Input: part model. Units: mm. Frame: model coordinates. A direction names the side the tool comes from. Round coordinates to 2 decimals unless told otherwise and drop trailing zeros. Loops run counter-clockwise (first coordinate to the right, second up) from the corner with the lowest first, then second, coordinate; pieces in that order, holes last. Notation, with made-up numbers: M 53.25,-6.5 L 82.25,-6.5 A11 cw 82.25,3.5 Z; hole C 51.5,0 d4. An arc over 180 degrees is marked long. Return JSON: item names as keys, results as strings. Group by question number.
1) Section C-C (x = -5.25). Output: boundary loops of the cut face in (y, z).
2) Material intervals for line 1 (X direction, y = -0.7, z = 4.75); line 2 (Z direction, x = 4.5, y = -1.4); line 3 (X direction, y = -0.7, z = -1), sorted ascending. Write a range as from..to.
3) Mould query, pull axis Z, two halves, no side actions, for faces 4 (the face through (7, -1, 10.412)), 5 (the face through (-4.957, -1, 4)), 6 (the face through (-13.082, -1, 8)). Classes: +Z half, -Z half, draft (parallel to the pull), parting line (faces both ways), or undercut.
4) Section D-D (z = 8.5). Output: boundary loops of the cut face in (x, y), plus the area to 3 significant figures.
5) Section B-B (z = 5.5). Output: boundary loops of the cut face in (x, y).
6) Section A-A (x = -7.75). Output: boundary loops of the cut face in (y, z), plus the area to 3 significant figures.
7) Access query for faces 1 (the face through (-12.7, -1, 5.987)), 2 (the face through (7.168, -1, -1)), 3 (the face through (1.418, -1, 0)). Directions: +Z, -Z, +X, -X, +Y, -Y. A direction counts if a zero-diameter tool reaches every point of the face in a straight line with its end or side. Return the directions, or none.
8) Contact query for flat-ended pins moving along their axis: P1, Ø1, axis at y = -1.5, z = 3, coming from the +X side; P2, Ø0.5, axis at y = -1, z = 3.5, coming from the -X side; P3, Ø1, axis at y = -1, z = 9, coming from the +X side. Output: stop coordinate, or through.
from build123d import *

# Parameters (mm, degrees)
F1_DEPTH = 2


with BuildPart() as f1:
    # F0 (on Front) → F1 (new body)
    with BuildSketch(Plane.XZ):
        Polygon((5.419874, 11.329587), (-11.338243, 11.329587), (-12.255757, 10.412073), (-13.082057, 10.412073), (-13.082057, 5.987073), (-12.25363, 5.987073), (-11.082057, 4.8155), (-11.082057, 3.158646), (-12.25363, 1.987073), (-13.082057, 1.987073), (-13.082057, -3.355442), (7.167943, -3.355442), (7.167943, 1.987073), (6.339516, 1.987073), (5.167943, 3.158646), (5.167943, 4.8155), (6.339516, 5.987073), (7.165815, 5.987073), (7.165815, 10.412073), (6.337388, 10.412073), align=None)
        Polygon((-12.082057, -1.183869), (-12.082057, 0.472986), (-10.910484, 1.644558), (-9.25363, 1.644558), (-8.082057, 0.472986), (-8.082057, -1.183869), (-9.25363, -2.355442), (-10.910484, -2.355442), align=None, mode=Mode.SUBTRACT)
        Polygon((-4.50363, 1.644558), (-3.332057, 0.472986), (-3.332057, -1.183869), (-4.50363, -2.355442), (-6.160484, -2.355442), (-7.332057, -1.183869), (-7.332057, 0.472986), (-6.160484, 1.644558), align=None, mode=Mode.SUBTRACT)
        Polygon((-8.082057, 9.158014), (-8.082057, 7.50116), (-9.25363, 6.329587), (-10.910484, 6.329587), (-12.082057, 7.50116), (-12.082057, 9.158014), (-10.910484, 10.329587), (-9.25363, 10.329587), align=None, mode=Mode.SUBTRACT)
        Polygon((-9.707057, 3.158646), (-9.707057, 4.8155), (-8.535484, 5.987073), (-6.87863, 5.987073), (-5.707057, 4.8155), (-5.707057, 3.158646), (-6.87863, 1.987073), (-8.535484, 1.987073), align=None, mode=Mode.SUBTRACT)
        Polygon((-7.332057, 9.158014), (-6.160484, 10.329587), (-4.50363, 10.329587), (-3.332057, 9.158014), (-3.332057, 7.50116), (-4.50363, 6.329587), (-6.160484, 6.329587), (-7.332057, 7.50116), align=None, mode=Mode.SUBTRACT)
        Polygon((0.24637, 1.644558), (1.417943, 0.472986), (1.417943, -1.183869), (0.24637, -2.355442), (-1.410484, -2.355442), (-2.582057, -1.183869), (-2.582057, 0.472986), (-1.410484, 1.644558), align=None, mode=Mode.SUBTRACT)
        Polygon((4.99637, 1.644558), (6.167943, 0.472986), (6.167943, -1.183869), (4.99637, -2.355442), (3.339516, -2.355442), (2.167943, -1.183869), (2.167943, 0.472986), (3.339516, 1.644558), align=None, mode=Mode.SUBTRACT)
        Polygon((-3.785484, 5.987073), (-2.12863, 5.987073), (-0.957057, 4.8155), (-0.957057, 3.158646), (-2.12863, 1.987073), (-3.785484, 1.987073), (-4.957057, 3.158646), (-4.957057, 4.8155), align=None, mode=Mode.SUBTRACT)
        Polygon((0.964516, 5.987073), (2.62137, 5.987073), (3.792943, 4.8155), (3.792943, 3.158646), (2.62137, 1.987073), (0.964516, 1.987073), (-0.207057, 3.158646), (-0.207057, 4.8155), align=None, mode=Mode.SUBTRACT)
        Polygon((-2.582057, 9.158014), (-1.410484, 10.329587), (0.24637, 10.329587), (1.417943, 9.158014), (1.417943, 7.50116), (0.24637, 6.329587), (-1.410484, 6.329587), (-2.582057, 7.50116), align=None, mode=Mode.SUBTRACT)
        Polygon((2.167943, 9.158014), (3.339516, 10.329587), (4.99637, 10.329587), (6.167943, 9.158014), (6.167943, 7.50116), (4.99637, 6.329587), (3.339516, 6.329587), (2.167943, 7.50116), align=None, mode=Mode.SUBTRACT)
    extrude(amount=F1_DEPTH)


solid = f1.part
Returned:
{
 "1": {"outline": "M -2,-3.36 L 0,-3.36 L 0,-2.36 L -2,-2.36 Z; M -2,1.64 L 0,1.64 L 0,6.33 L -2,6.33 Z; M -2,10.33 L 0,10.33 L 0,11.33 L -2,11.33 Z"},
 "2": {"line 1": "x = -11.08..-9.71, -5.71..-4.96, -0.96..-0.21, 3.79..5.17", "line 2": "z = -3.36..-2.36, 1.64..6.33, 10.33..11.33", "line 3": "x = -13.08..-12.08, -8.08..-7.33, -3.33..-2.58, 1.42..2.17, 6.17..7.17"},
 "3": {"face 4": "+Z half", "face 5": "undercut", "face 6": "draft"},
 "4": {"outline": "M -13.08,-2 L -12.08,-2 L -12.08,0 L -13.08,0 Z; M -8.08,-2 L -7.33,-2 L -7.33,0 L -8.08,0 Z; M -3.33,-2 L -2.58,-2 L -2.58,0 L -3.33,0 Z; M 1.42,-2 L 2.17,-2 L 2.17,0 L 1.42,0 Z; M 6.17,-2 L 7.17,-2 L 7.17,0 L 6.17,0 Z", "area": "8.50 mm^2"},
 "5": {"outline": "M -11.77,-2 L -9.02,-2 L -9.02,0 L -11.77,0 Z; M -6.39,-2 L -4.27,-2 L -4.27,0 L -6.39,0 Z; M -1.64,-2 L 0.48,-2 L 0.48,0 L -1.64,0 Z; M 3.11,-2 L 5.85,-2 L 5.85,0 L 3.11,0 Z"},
 "6": {"outline": "M -2,-3.36 L 0,-3.36 L 0,1.99 L -2,1.99 Z; M -2,5.99 L 0,5.99 L 0,11.33 L -2,11.33 Z", "area": "21.4 mm^2"},
 "7": {"face 1": "-X, +Y, -Y", "face 2": "+Z, -Z, +X, +Y, -Y", "face 3": "+Y, -Y"},
 "8": {"P1": "stops at x = 5.83", "P2": "stops at x = -11.08", "P3": "stops at x = 7.17"}
}
